Check sheet for the modelled part. Datum: model origin and axes. Units: mm. Face numbers are marked on the shaded views. A direction names the side the tool comes from. Round coordinates to 2 decimals unless told otherwise and drop trailing zeros. Write each loop counter-clockwise with the first axis right and the second up, starting at its lowest first coordinate (ties: lowest second). Pieces come first, ordered by that corner, then holes.
Item 1: Material ranges on line 1 along Y through (x, z) = (-1, 11); line 2 along Y through (x, z) = (-1, 5.5); line 3 along X through (y, z) = (-14, 12.5), recorded low to high.
Item 2: Depth check by flat-ended pin: pin 1 (6 mm diameter, centred on x = -35, y = 15.5, fed in from +Z); pin 2 (8 mm diameter, centred on y = -34.5, z = 31.5, fed in from -X); pin 3 (12 mm diameter, centred on y = -30, z = 6, fed in from +X). Enter the tip coordinate at first touch or a pass-through.
Item 3: Section check D-D, the plane z = 33.5. Record the cut outline in (x, y).
Item 4: Set-up check for the marked faces 1, 2 and 3: record each of +Z, -Z, +X, -X, +Y, -Y from which the full face is reachable in a straight line by a thin tool's end or side.
Item 5: Release check for a two-part mould opening along Y. For the marked faces 4 and 5 record: pulls with the +Y half, pulls with the -Y half, needs draft (parallel to the pull), parting line crosses it, or undercut.
Item 6: Section check C-C, the plane z = 25.5. Record the cut outline in (x, y).
from build123d import *

# Parameters (mm, degrees)
F0_R     = 40
F0_R_2   = 38
F1_DEPTH = 15
F2_W     = 2
F2_H     = 5.6
F5_W     = 12
F5_H     = 12
F6_DEPTH = 5
F7_SIZE  = 1.19999


# Not quite as in the source:
# - a fillet or chamfer is up to 0.001 mm smaller than in the source, because OpenCascade refuses the exact size


with BuildPart() as f1:
    # F0 (on Top) → F1 (new body)
    with BuildSketch(Plane.XY):
        Circle(F0_R)
        Circle(F0_R_2, mode=Mode.SUBTRACT)
    extrude(amount=F1_DEPTH)

    # F2 (on Front) → F3 (revolve, cut)
    with BuildSketch(Plane.XZ):
        with Locations((38.2, 2.8)):
            Rectangle(F2_W, F2_H)
        Polygon((45, 30), (38, 15), (40, 15), (47.4, 30), (47.4, 45), (45, 45), align=None)
    revolve(axis=Axis((0, 0, 15), (0, 0, 1)), mode=Mode.SUBTRACT)

    # F2 (on Front) → F4 (revolve)
    with BuildSketch(Plane.XZ):
        Polygon((45, 30), (38, 15), (40, 15), (47.4, 30), (47.4, 45), (45, 45), align=None)
    revolve(axis=Axis((0, 0, 15), (0, 0, 1)))

    # F5 (on face) → F6 (cut)
    with BuildSketch(Plane.XY.offset(45)):
        with Locations((0, 46)):
            Rectangle(F5_W, F5_H)
        Polygon((-15.5538475773, 37.4400542571), (-21.5538475773, 47.8323591025), (-31.9461524227, 41.8323591025), (-25.9461524227, 31.4400542571), align=None)
        Polygon((-32.9400542571, 24.4461524227), (-43.3323591025, 30.4461524227), (-49.3323591025, 20.0538475773), (-38.9400542571, 14.0538475773), align=None)
        with Locations((-47.5, -1.5)):
            Rectangle(F5_W, F5_H)
        Polygon((-38.9400542571, -17.0538475773), (-49.3323591025, -23.0538475773), (-43.3323591025, -33.4461524227), (-32.9400542571, -27.4461524227), align=None)
        Polygon((-25.9461524227, -34.4400542571), (-31.9461524227, -44.8323591025), (-21.5538475773, -50.8323591025), (-15.5538475773, -40.4400542571), align=None)
        with Locations((0, -49)):
            Rectangle(F5_W, F5_H)
        Polygon((15.5538475773, -40.4400542571), (21.5538475773, -50.8323591025), (31.9461524227, -44.8323591025), (25.9461524227, -34.4400542571), align=None)
        Polygon((32.9400542571, -27.4461524227), (43.3323591025, -33.4461524227), (49.3323591025, -23.0538475773), (38.9400542571, -17.0538475773), align=None)
        with Locations((47.5, -1.5)):
            Rectangle(F5_W, F5_H)
        Polygon((38.9400542571, 14.0538475773), (49.3323591025, 20.0538475773), (43.3323591025, 30.4461524227), (32.9400542571, 24.4461524227), align=None)
        Polygon((25.9461524227, 31.4400542571), (31.9461524227, 41.8323591025), (21.5538475773, 47.8323591025), (15.5538475773, 37.4400542571), align=None)
    extrude(amount=-F6_DEPTH, mode=Mode.SUBTRACT)

    # F7 (size 1.2 in the source; OpenCascade refuses exactly that, so slightly less here)
    f7_edges = [f1.edges().sort_by_distance(p)[0] for p in [
        (-38, 0, 5.6),
    ]]
    chamfer(f7_edges, length=F7_SIZE)


solid = f1.part
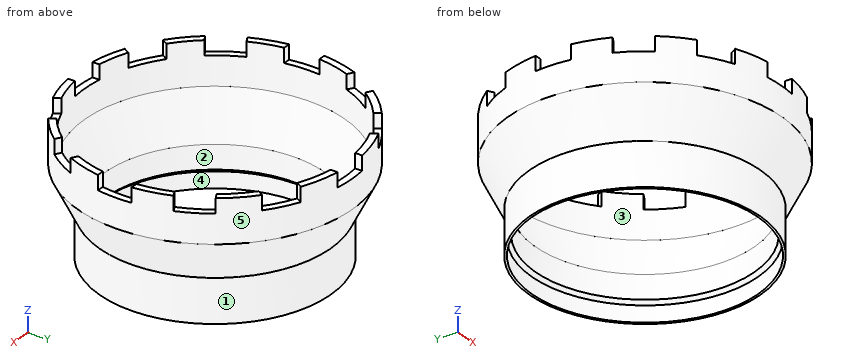
Values found:
1. line 1: y = -39.99 to -37.99, 37.99 to 39.99
1. line 2: y = -39.99 to -39.19, 39.19 to 39.99
1. line 3: x = -37.47 to -35.33, 35.33 to 37.47
2. pin 1: stops at z = 22.03
2. pin 2: stops at x = -36.28
2. pin 3: stops at x = 32
3. outline: circle Ø94.8 at (0, 0); hole circle Ø90 at (0, 0)
4. face 1: -Z
4. face 2: +Z, -Z
4. face 3: +Z
5. face 4: undercut
5. face 5: parting line crosses it
6. outline: circle Ø90.36 at (0, 0); hole circle Ø85.8 at (0, 0)
